from build123d import *

# Parameters (mm, degrees)
F0_W     = 49
F0_H     = 46.5
F1_DEPTH = 10
F2_R     = 2
F3_DEPTH = 10.001
F4_R     = 2
F5_DEPTH = 20
F6_R     = 2
F7_DEPTH = 20


with BuildPart() as f1:
    # F0 (on Front) → F1 (new body)
    with BuildSketch(Plane.XZ):
        with Locations((0, 23.25)):
            Rectangle(F0_W, F0_H)
    extrude(amount=F1_DEPTH)

    # F2 (on face) → F3 (cut, through all)
    with BuildSketch(Plane(origin=(0, 0, 0), x_dir=(-1, 0, 0), z_dir=(0, 1, 0))):
        with Locations((-12.25, 5)):
            Circle(F2_R)
        with Locations((7.75, 5)):
            Circle(F2_R)
    extrude(amount=-F3_DEPTH, mode=Mode.SUBTRACT)

    # F4 (on face) → F5 (cut)
    with BuildSketch(Plane.XY.offset(46.5)):
        with Locations((16.5, -5)):
            Circle(F4_R)
        with Locations((-16.5, -5)):
            Circle(F4_R)
    extrude(amount=-F5_DEPTH, mode=Mode.SUBTRACT)

    # F6 (on face) → F7 (cut)
    with BuildSketch(Plane(origin=(0, 0, 0), x_dir=(1, 0, 0), z_dir=(0, 0, -1))):
        with Locations((-16.5, 5)):
            Circle(F6_R)
        with Locations((16.5, 5)):
            Circle(F6_R)
    extrude(amount=-F7_DEPTH, mode=Mode.SUBTRACT)


solid = f1.part
Could you check a few things on this model? Use its own coordinates, in mm. A direction names the side the tool comes from. Round coordinates to 2 decimals unless told otherwise and drop trailing zeros. Order: outer loops, then holes, each group sorted by start corner. A loop starts at its lowest first (then second) coordinate and runs counter-clockwise, first axis right, second up.
Q1. Imagine slicing it at A-A, the plane z = 5. List the corners of the cut face in (x, y) for me, then the cut area to 3 significant figures.
Geometry says:
outline: (-24.5, -10) - (-9.75, -10) - (-9.75, 0) - (-24.5, 0) - close; (-5.75, -10) - (10.25, -10) - (10.25, 0) - (-5.75, 0) - close; (14.25, -10) - (24.5, -10) - (24.5, 0) - (14.25, 0) - close; hole circle Ø4 at (-16.5, -5); hole circle Ø4 at (16.5, -5)
area: 385 mm2
Q2. Please list where these lines run through material, in increasing order: probe 1 along X at (y, z) = (-5.75, 9); probe 2 along Z at (x, y) = (-7.75, -5); probe 3 along X at (y, z) = (-5.25, 14.5).
Geometry says:
probe 1: x = -24.5 to -18.35, -14.65 to 14.65, 18.35 to 24.5
probe 2: z = 0 to 3, 7 to 46.5
probe 3: x = -24.5 to -18.48, -14.52 to 14.52, 18.48 to 24.5
Q3. Imagine slicing it at D-D, the plane x = 16.5. List the corners of the cut face in (y, z) for me.
Geometry says:
outline: (-10, 0) - (-7, 0) - (-7, 20) - (-3, 20) - (-3, 0) - (0, 0) - (0, 46.5) - (-3, 46.5) - (-3, 26.5) - (-7, 26.5) - (-7, 46.5) - (-10, 46.5) - close
Q4. Imagine slicing it at B-B, the plane x = -7.5. List the corners of the cut face in (y, z) for me.
Geometry says:
outline: (-10, 0) - (0, 0) - (0, 3.02) - (-10, 3.02) - close; (-10, 6.98) - (0, 6.98) - (0, 46.5) - (-10, 46.5) - close
Q5. I'm going to push flat-ended pins straight in: P1, Ø2.5, axis at x = 16.5, y = -5, coming from the -Z side; P2, Ø3.5, axis at x = 12.25, z = 5, coming from the +Y side. Where does each tip first touch, or does it pass through?
Geometry says:
P1: stops at z = 20
P2: passes through
Q6. Thinking about a two-plate mould opening in X: for faces 4 (the face through (24.5, -5, 23)), 5 (the face through (-18.1, -6.2, 36.6)), 6 (the face through (0, -10, 24)), 7 (the face through (16, -5, 26.5)), which applies, released by +X, released by -X, zero draft, split by the parting line, or undercut?
Geometry says:
face 4: released by +X
face 5: undercut
face 6: zero draft
face 7: undercut
Q7. Imagine slicing it at C-C, the plane z = 32. List the corners of the cut face in (x, y) for me.
Geometry says:
outline: (-24.5, -10) - (24.5, -10) - (24.5, 0) - (-24.5, 0) - close; hole circle Ø4 at (-16.5, -5); hole circle Ø4 at (16.5, -5)
Q8. Which directions (+Z, -Z, +X, -X, +Y, -Y) give clear straight access to the entire face, cutting with the end or side of a thin tool? Please do faces 1 (the face through (0, -5, 46.5)), 2 (the face through (-17, -5, 26.5)), 3 (the face through (-18.498, -5.088, 9.86)).
Geometry says:
face 1: +Z, +X, -X, +Y, -Y
face 2: +Z
face 3: -Z
